```python
from build123d import *

# Parameters (mm, degrees)
SKETCH2_W           = 720
SKETCH2_H           = 720
SKETCH2_R           = 30
BOSS_EXTRUDE1_DEPTH = 2
SKETCH3_R           = 5
BOSS_EXTRUDE2_DEPTH = 2


with BuildPart() as part:
    # Sketch2 → Boss-Extrude1 (new body)
    with BuildSketch(Plane.XY):
        Rectangle(SKETCH2_W, SKETCH2_H)
        Circle(SKETCH2_R, mode=Mode.SUBTRACT)
    extrude(amount=BOSS_EXTRUDE1_DEPTH)

    # Sketch3 → Boss-Extrude2 (add)
    with BuildSketch(Plane.XY.offset(2)):
        with Locations((0, 340)):
            Circle(SKETCH3_R)
        with Locations((-340, 0)):
            Circle(SKETCH3_R)
        with Locations((0, -340)):
            Circle(SKETCH3_R)
        with Locations((340, 0)):
            Circle(SKETCH3_R)
    extrude(amount=BOSS_EXTRUDE2_DEPTH)


solid = part.part
```
Verification items for the finished model (mm, model axes). Give positions to 0.01 mm unless a question says otherwise; leave off trailing zeros. Write each loop counter-clockwise with the first axis right and the second up, starting at its lowest first coordinate (ties: lowest second). Pieces come first, ordered by that corner, then holes. Notation, with made-up numbers: (80.25, -23) - (96.25, -23) arc R19 ccw to (96.25, 8) - close; hole circle Ø4 at (29, 44.25). An arc over 180 degrees is marked (long way). Put each result on its own line as item: value.
Q1. Section check A-A on z = 3.1. Record the cut outline in (x, y), and give its area (3 significant figures).
Result:
outline: circle Ø10 at (-340, 0); circle Ø10 at (0, -340); circle Ø10 at (0, 340); circle Ø10 at (340, 0)
area: 314 mm2
Q2. Mould release check, pull along Y, two halves, no side actions. Record for faces 1 (the face through (-29.97, 1.32, 0.99)), 2 (the face through (-5, 85, 0)): released by +Y, released by -Y, zero draft, split by the parting line, or undercut.
Result:
face 1: undercut
face 2: zero draft
Q3. Scan lines: probe 1 along Y at (x, z) = (0, 1.3); probe 2 along Z at (x, y) = (64.5, -303). Record each from-to range of solid material in increasing order. Write a range as from..to.
Result:
probe 1: -360..-30, 30..360
probe 2: 0..2
Q4. Depth check by flat-ended pin: P1, Ø10, axis at x = 100.5, y = 103, coming from the -Z side. Enter the tip coordinate at first touch or a pass-through.
Result:
P1: z = 0
Q5. Section check B-B on x = -184.5. Record the cut outline in (y, z).
Result:
outline: (-360, 0) - (360, 0) - (360, 2) - (-360, 2) - close
